Source: CAD feature listing. Evaluate the final solid. Frame: model axes, mm. Coordinates: 2 decimals unless noted, no trailing zeros. Loops run counter-clockwise (first coordinate to the right, second up) from the corner with the lowest first, then second, coordinate; pieces in that order, holes last.
from build123d import *

# Parameters (mm, degrees)
SKETCH1_W           = 114.3
SKETCH1_H           = 139.7
BOSS_EXTRUDE1_DEPTH = 3.18
SKETCH2_R           = 1.5
SKETCH2_W           = 3.18
SKETCH2_H           = 59.975
CUT_EXTRUDE1_DEPTH  = 91.306463778
CUT_EXTRUDE5_DEPTH  = 12
SKETCH5_R           = 32.671394307
CUT_EXTRUDE6_DEPTH  = 10
SKETCH9_R           = 1.042012373
CUT_EXTRUDE8_DEPTH  = 91.306463778


with BuildPart() as part:
    # Sketch1 → Boss-Extrude1 (new body)
    with BuildSketch(Plane.XY):
        Rectangle(SKETCH1_W, SKETCH1_H)
    extrude(amount=BOSS_EXTRUDE1_DEPTH)

    # Sketch2 → Cut-Extrude1 (cut, through all)
    with BuildSketch(Plane.XY.offset(3.18)):
        with Locations((-55.15, 0)):
            Circle(SKETCH2_R)
        with Locations((55.15, 0)):
            Circle(SKETCH2_R)
        Polygon((-10, 69.85), (10, 69.85), (10, 66.67), (1.5, 66.67), (1.5, 62.67), (3.5, 62.67), (3.5, 59.67), (1.5, 59.67), (1.5, 56.67), (-1.5, 56.67), (-1.5, 59.67), (-3.5, 59.67), (-3.5, 62.67), (-1.5, 62.67), (-1.5, 66.67), (-10, 66.67), align=None)
        Polygon((-10, -69.85), (-10, -66.67), (-1.5, -66.67), (-1.5, -62.67), (-3.5, -62.67), (-3.5, -59.67), (-1.5, -59.67), (-1.5, -56.67), (1.5, -56.67), (1.5, -59.67), (3.5, -59.67), (3.5, -62.67), (1.5, -62.67), (1.5, -66.67), (10, -66.67), (10, -69.85), align=None)
        with Locations((-55.56, 39.8625)):
            Rectangle(SKETCH2_W, SKETCH2_H)
        with Locations((-55.56, -39.8625)):
            Rectangle(SKETCH2_W, SKETCH2_H)
        with Locations((55.56, -39.8625)):
            Rectangle(SKETCH2_W, SKETCH2_H)
        with Locations((55.56, 39.8625)):
            Rectangle(SKETCH2_W, SKETCH2_H)
    extrude(amount=-CUT_EXTRUDE1_DEPTH, mode=Mode.SUBTRACT)

    # Sketch4 → Cut-Extrude5 (cut)
    with BuildSketch(Plane.XY):
        with BuildLine():
            Line((-25.57107609, -41.8625), (-45.57107609, -41.8625))
            Line((-45.57107609, -41.8625), (-45.57107609, -45.3625))
            Line((-45.57107609, -45.3625), (-48.57107609, -45.3625))
            Line((-48.57107609, -45.3625), (-48.57107609, -34.3625))
            Line((-48.57107609, -34.3625), (-45.57107609, -34.3625))
            Line((-45.57107609, -34.3625), (-45.57107609, -37.8625))
            Line((-45.57107609, -37.8625), (-31.57107609, -37.8625))
            Line((-31.57107609, -37.8625), (-31.57107609, -33.087601989))
            Line((-31.57107609, -33.087601989), (-28.57107609, -33.087601989))
            ThreePointArc((-28.57107609, -33.087601989), (-27.787526444, -36.79230316), (-25.57107609, -39.8625))
            Line((-25.57107609, -39.8625), (-25.57107609, -41.8625))
        make_face()
    extrude(amount=CUT_EXTRUDE5_DEPTH, mode=Mode.SUBTRACT)

    # Sketch5 → Cut-Extrude6 (cut)
    with BuildSketch(Plane.XY.offset(3.18)):
        with Locations((11.462576996, 0)):
            Circle(SKETCH5_R)
    extrude(amount=-CUT_EXTRUDE6_DEPTH, mode=Mode.SUBTRACT)

    # Sketch9 → Cut-Extrude8 (cut, through all)
    with BuildSketch(Plane.XY.offset(3.18)):
        with Locations((37.991387583, -21.1)):
            Circle(SKETCH9_R)
        with Locations((37.991387583, 21.008299604)):
            Circle(SKETCH9_R)
    extrude(amount=-CUT_EXTRUDE8_DEPTH, mode=Mode.SUBTRACT)


solid = part.part
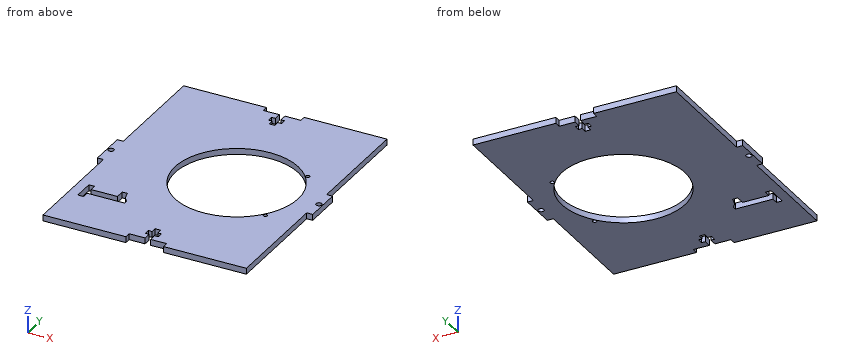
Q1. Line query: line 1 along Y through (x, z) = (-55.15, 2.4) (3 decimals); line 2 along X through (y, z) = (59, 2.85); line 3 along X through (y, z) = (-44, 2.6). Output: solid intervals per line, ascending.
Q2. Section D-D, the plane z = 1.4. Count the separate pieces of the cut face and the enclosed holes in it, plus the area to 3 significant figures.
Q3. Contact query for flat-ended pins moving along their axis: pin 1 Ø1.5 at (y, z) = (58, 1.5) entering from +X; pin 2 Ø1.6 at (x, z) = (-55, 1.5) entering from -Y (3 decimals); pin 3 Ø1.5 at (y, z) = (21, 0.5) entering from -X. Output: stop coordinate, or through.
Q4. Section C-C, the plane y = -25. Return the cut outline in (x, z), plus the area to 3 significant figures.
Q5. Section A-A, the plane x = -42. Return the cut outline in (y, z).
Q6. Section B-B, the plane y = 0. Return the cut outline in (x, z), plus the area to 3 significant figures.
Derived:
1. line 1: y = -9.875 to -1.5, 1.5 to 9.875
1. line 2: x = -53.97 to -1.5, 1.5 to 53.97
1. line 3: x = -53.97 to -48.57, -45.57 to 53.97
2. separate pieces: 1
2. enclosed holes: 6
2. area: 11,500 mm2
3. pin 1: stops at x = 53.97
3. pin 2: stops at y = -9.875
3. pin 3: stops at x = -53.97
4. outline: (-53.97, 0) - (-9.57, 0) - (-9.57, 3.18) - (-53.97, 3.18) - close; (32.5, 0) - (53.97, 0) - (53.97, 3.18) - (32.5, 3.18) - close
4. area: 209 mm2
5. outline: (-69.85, 0) - (-41.86, 0) - (-41.86, 3.18) - (-69.85, 3.18) - close; (-37.86, 0) - (69.85, 0) - (69.85, 3.18) - (-37.86, 3.18) - close
6. outline: (-57.15, 0) - (-56.65, 0) - (-56.65, 3.18) - (-57.15, 3.18) - close; (-53.65, 0) - (-21.21, 0) - (-21.21, 3.18) - (-53.65, 3.18) - close; (44.13, 0) - (53.65, 0) - (53.65, 3.18) - (44.13, 3.18) - close; (56.65, 0) - (57.15, 0) - (57.15, 3.18) - (56.65, 3.18) - close
6. area: 137 mm2
